from build123d import *

# Parameters (mm, degrees)
SKETCH_1_W          = 42
SKETCH_1_H          = 26
EXTRUDE_1_DEPTH     = 10
SKETCH_2_R          = 4
CUT_EXTRUDE_1_DEPTH = 5
FILLET_1_R          = 3


with BuildPart() as part:
    # 草图1 → 凸台-拉伸1 (new body)
    with BuildSketch(Plane(origin=(0, 0, 0), x_dir=(1, 0, 0), z_dir=(0, 1, 0))):
        Rectangle(SKETCH_1_W, SKETCH_1_H)
    extrude(amount=EXTRUDE_1_DEPTH)

    # 草图2 → 切除-拉伸1 (cut)
    with BuildSketch(Plane(origin=(0, 10, 0), x_dir=(1, 0, 0), z_dir=(0, 1, 0))):
        with Locations(Location((-0.035567837, 4.026194604, 0), (0, 0, 270))):
            Circle(SKETCH_2_R)
    extrude(amount=-CUT_EXTRUDE_1_DEPTH, mode=Mode.SUBTRACT)

    # 圆角1
    fillet_1_edges = [part.edges().sort_by_distance(p)[0] for p in [
        (21, 5, 13),
        (21, 5, -13),
    ]]
    fillet(fillet_1_edges, radius=FILLET_1_R)


solid = part.part
Can you work these out from the model? Positions are in its coordinate system, mm. Round coordinates to 2 decimals unless told otherwise and drop trailing zeros. Loops run counter-clockwise (first coordinate to the right, second up) from the corner with the lowest first, then second, coordinate; pieces in that order, holes last. Notation, with made-up numbers: (25, 46.5) - (48, 46.5) arc R24 cw to (48, 67.5) - close; hole circle Ø7 at (-31, 2.5). An arc over 180 degrees is marked (long way). Write item = value, one per line. Start each with the question number.
(1) If we mould it in two halves opening along X, with no side actions, what happens to faces 1 (the face through (0, 5, -4)), 2 (the face through (-2.47, 7.54, -7.2)), 3 (the face through (21, 5, 0)), 4 (the face through (0, 0, 0))? For each: released by +X, released by -X, zero draft, split by the parting line, or undercut.
(2) If we section it at B-B (y = 5.75): Please give me the cut outline in (x, z).
(3) If I drill on probe 1 along Z at (x, y) = (-1, 8); probe 2 along X at (y, z) = (9.5, -5.5); probe 3 along X at (y, z) = (9.25, -0.5), over which ranges is the centre line in solid material (lowest first)? Write a range as [from, to].
(4) For P1, Ø4, axis at x = -1, z = -3.5, coming from the +Y side, with a flat end and sliding along its axis, tell me the tip position at first contact or that it passes through.
(5) If we section it at C-C (x = 2): Please give me the cut outline in (y, z), and give its area (3 significant figures).
(6) If we section it at A-A (z = -0.75): Please give me the cut outline in (x, y).
Ans:
q1.face_1 = undercut
q1.face_2 = undercut
q1.face_3 = released by +X
q1.face_4 = zero draft
q2.outline = (-21, -13) - (18, -13) arc R3 ccw to (21, -10) - (21, 10) arc R3 ccw to (18, 13) - (-21, 13) - close; hole circle Ø8 at (-0.04, -4.03)
q3.probe_1 = [-13, -7.91], [-0.14, 13]
q3.probe_2 = [-21, -3.75], [3.68, 21]
q3.probe_3 = [-21, -1.92], [1.85, 21]
q4.P1 = 5
q5.outline = (0, -13) - (10, -13) - (10, -7.47) - (5, -7.47) - (5, -0.58) - (10, -0.58) - (10, 13) - (0, 13) - close
q5.area = 226 mm²
q6.outline = (-21, 0) - (21, 0) - (21, 10) - (2.26, 10) - (2.26, 5) - (-2.33, 5) - (-2.33, 10) - (-21, 10) - close
